from build123d import *

# Parameters (mm, degrees)
SKETCH1_R           = 20
BOSS_EXTRUDE1_DEPTH = 25
CHAMFER1_SIZE       = 10
SKETCH2_R           = 2.5
CUT_EXTRUDE1_DEPTH  = 15
SKETCH3_R           = 7.5
BOSS_EXTRUDE2_DEPTH = 7


with BuildPart() as part:
    # Sketch1 → Boss-Extrude1 (new body)
    with BuildSketch(Plane.XY):
        Circle(SKETCH1_R)
    extrude(amount=BOSS_EXTRUDE1_DEPTH)

    # Chamfer1
    chamfer1_edges = [part.edges().sort_by_distance(p)[0] for p in [
        (-20, 0, 25),
    ]]
    chamfer(chamfer1_edges, length=CHAMFER1_SIZE)

    # Sketch2 → Cut-Extrude1 (cut)
    with BuildSketch(Plane.XY.offset(25)):
        Circle(SKETCH2_R)
    extrude(amount=-CUT_EXTRUDE1_DEPTH, mode=Mode.SUBTRACT)

    # Sketch3 → Boss-Extrude2 (add)
    with BuildSketch(Plane(origin=(0, 0, 0), x_dir=(-1, 0, 0), z_dir=(0, 0, -1))):
        Circle(SKETCH3_R)
    extrude(amount=BOSS_EXTRUDE2_DEPTH)


solid = part.part
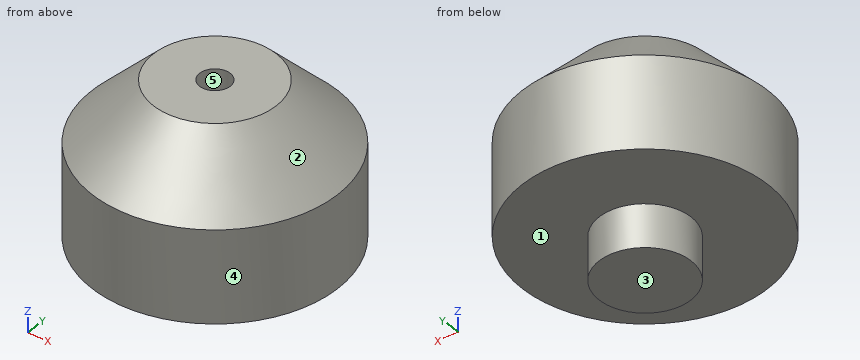
Part model, mm, in its own coordinate system. Face numbers are marked on the shaded views. A direction names the side the tool comes from. Give positions to 0.01 mm unless a question says otherwise; leave off trailing zeros. Write each loop counter-clockwise with the first axis right and the second up, starting at its lowest first coordinate (ties: lowest second). Pieces come first, ordered by that corner, then holes.
1) Cut at C-C on z = -5. Write the cut outline in (x, y).
Resolved:
outline: circle Ø15 at (0, 0)
2) Cut at D-D on z = 2. Write the cut outline in (x, y).
Resolved:
outline: circle Ø40 at (0, 0)
3) Pin check, flat tips, straight feed: pin 1 (2 mm diameter, centred on y = -16, z = 7, fed in from +X); pin 2 (3 mm diameter, centred on y = -7, z = 5.5, fed in from -X); pin 3 (6 mm diameter, centred on y = 7.5, z = 13.5, fed in from +X). Stop position of each tip, or through.
Resolved:
pin 1: stops at x = 13.23
pin 2: stops at x = -19.23
pin 3: stops at x = 19.49
4) Probe L1, parallel to Y at x = 0, z = 14; L2, parallel to Z at x = 8.5, y = -3.5; L3, parallel to Y at x = 0, z = 20. List the from-to ranges inside material, lowest first.
Resolved:
L1: y = -20 to -2.5, 2.5 to 20
L2: z = 0 to 25
L3: y = -15 to -2.5, 2.5 to 15
5) Which spindle directions (+Z, -Z, +X, -X, +Y, -Y) get a long thin tool onto all of the face, cutting with end or side? Do the marked faces 1 and 2. Say none if no direction does.
Resolved:
face 1: -Z
face 2: +Z
6) Two-plate mould, pull along Y, no slides. Class the marked faces 3, 4 and 5: released by +Y, released by -Y, zero draft, split by the parting line, or undercut.
Resolved:
face 3: zero draft
face 4: split by the parting line
face 5: undercut
7) Cut at A-A on x = 0. Write the cut outline in (y, z).
Resolved:
outline: (-20, 0) - (-7.5, 0) - (-7.5, -7) - (7.5, -7) - (7.5, 0) - (20, 0) - (20, 15) - (10, 25) - (2.5, 25) - (2.5, 10) - (-2.5, 10) - (-2.5, 25) - (-10, 25) - (-20, 15) - close
